from build123d import *

# Parameters (mm, degrees)
SKETCH1_R           = 35
BOSS_EXTRUDE1_DEPTH = 35
SKETCH2_R           = 25
BOSS_EXTRUDE2_DEPTH = 65
SKETCH5_R           = 26
SKETCH7_R           = 6.5
SKETCH6_R           = 21
SKETCH8_R           = 6.5
SKETCH13_R          = 6.5
CUT_EXTRUDE2_DEPTH  = 100


with BuildPart() as part:
    # Sketch1 → Boss-Extrude1 (new body)
    with BuildSketch(Plane(origin=(0, 0, 0), x_dir=(0, 0, -1), z_dir=(1, 0, 0))):
        Circle(SKETCH1_R)
    extrude(amount=BOSS_EXTRUDE1_DEPTH)

    # Sketch2 → Boss-Extrude2 (add)
    with BuildSketch(Plane(origin=(35, 0, 0), x_dir=(0, 0, -1), z_dir=(1, 0, 0))):
        Circle(SKETCH2_R)
    extrude(amount=BOSS_EXTRUDE2_DEPTH)

    # Sketch5 → Cut-Loft1 section 0
    with BuildSketch(Plane.ZY):
        Circle(SKETCH5_R)
    # Sketch7 → Cut-Loft1 section 1
    with BuildSketch(Plane.ZY.offset(-30.8)):
        Circle(SKETCH7_R)
    loft(mode=Mode.SUBTRACT)

    # Sketch6 → Cut-Loft2 section 0
    with BuildSketch(Plane(origin=(100, 0, 0), x_dir=(0, 0, -1), z_dir=(1, 0, 0))):
        Circle(SKETCH6_R)
    # Sketch8 → Cut-Loft2 section 1
    with BuildSketch(Plane(origin=(31.8, 0, 0), x_dir=(0, 0, -1), z_dir=(1, 0, 0))):
        Circle(SKETCH8_R)
    loft(mode=Mode.SUBTRACT)

    # Sketch12 → Cut-Revolve1 (revolve, cut)
    with BuildSketch(Plane.XY, mode=Mode.PRIVATE) as cut_revolve1_sk:
        Polygon((0, 35), (5, 35), (5, 32), (8, 32), (8, 35), (13, 35), (13, 32), (16, 32), (16, 35), (16, 38.455510313), (0, 38.455510313), align=None)
    revolve(cut_revolve1_sk.sketch.rotate(Axis((0, 0, 0), (1, 0, 0)), 90), axis=Axis((0, 0, 0), (1, 0, 0)), mode=Mode.SUBTRACT)

    # Sketch13 → Cut-Extrude2 (cut)
    with BuildSketch(Plane.ZY):
        Circle(SKETCH13_R)
    extrude(amount=-CUT_EXTRUDE2_DEPTH, mode=Mode.SUBTRACT)


solid = part.part
Can you work these out from the model? Positions are in its coordinate system, mm. A direction names the side the tool comes from. Coordinates: 2 decimals unless noted, no trailing zeros. Loops run counter-clockwise (first coordinate to the right, second up) from the corner with the lowest first, then second, coordinate; pieces in that order, holes last. Notation, with made-up numbers: (47.5, -12) - (92.5, -12) arc R29 ccw to (92.5, 17) - close; hole circle Ø5 at (58.25, -24.5). An arc over 180 degrees is marked (long way). Answer as a JSON object with one key per item and string values. Group by question number.
Item 1: If I drill on L1, parallel to X at y = 26, z = 22.5; L2, parallel to Y at x = 31.65, z = 0, over which ranges is the centre line in solid material (lowest first)? Write a range as from..to.
Item 2: If we mould it in two halves opening along Z, with no side actions, what happens to faces 1 (the face through (5, 28.4, 15.4)), 2 (the face through (14.52, 31.24, -6.94)), 3 (the face through (31.293, -3.955, -5.158))? For each: released by +Z, released by -Z, zero draft, split by the parting line, or undercut.
Item 3: If we section it at C-C (x = 82): List the corners of the cut face in (y, z) for me.
Item 4: If we section it at B-B (x = 37): List the corners of the cut face in (y, z) for me.
Item 5: On a 3-axis mill with a long thin cutter (end or side, diameter ignored), from which of +Z, -Z, +X, -X, +Y, -Y can I reach the whole of each face in a straight line? I mean faces 4 (the face through (100, 20.5, 5.7)), 5 (the face through (16, 28.4, -15.4)), 6 (the face through (35, 8, 24)). Say none if no direction works.
Item 6: For pin 1 (5 mm diameter, centred on x = 40, z = -15, fed in from +Y); pin 2 (12 mm diameter, centred on x = 18.5, z = -23, fed in from -Y); pin 3 (1 mm diameter, centred on x = 32, z = -26, fed in from +Y), each with a flat end and sliding along its axis, tell me the tip position at first contact or that it passes through.
Returned:
{
 "1": {"L1": "x = 0..5, 8..13, 16..35", "L2": "y = -35..-6.5, 6.5..35"},
 "2": {"face 1": "zero draft", "face 2": "split by the parting line", "face 3": "undercut"},
 "3": {"outline": "circle Ø50 at (0, 0); hole circle Ø34.35 at (0, 0)"},
 "4": {"outline": "circle Ø50 at (0, 0); hole circle Ø15.21 at (0, 0)"},
 "5": {"face 4": "+Z, -Z, +X, +Y, -Y", "face 5": "none", "face 6": "+X"},
 "6": {"pin 1": "stops at y = 21.65", "pin 2": "stops at y = -30.59", "pin 3": "stops at y = 23.97"}
}
